```python
from build123d import *

# Parameters (mm, degrees)
F0_W         = 77.8764
F0_H         = 158.496
F1_DEPTH     = 7.2898
F2_R         = 9.525
F3_R         = 5.7077755574
F4_DEPTH     = 0.127
F5_W         = 9.2544863001
F5_H         = 0.6169676781
F6_DEPTH     = 0.381
F8_DEPTH     = 0.635
F9_R         = 1.016
F10_R        = 1.9930126565
F11_DEPTH    = 12.7
F13_W        = 8.6497310549
F13_H        = 2.2564521059
F14_DEPTH    = 12.7
F16_DEPTH    = 2.159
F18_DEPTH    = 0.635
F19_T1_DEPTH = 2.8833260431
F19_T3_DEPTH = 2.8575
F19_T5_DEPTH = 2.8319706152
F21_DEPTH    = 0.635
F22_T1_DEPTH = 3.4834715988
F22_T3_DEPTH = 3.4925
F22_T5_DEPTH = 3.5015570173
F23_R        = 0.635


# Not quite as in the source:
# - a fillet or chamfer that OpenCascade refuses, or shapes differently, is made with other operations: its cross-section is extruded or revolved along the edge and cut away or added


with BuildPart() as f1:
    # F0 (on Front) → F1 (new body)
    with BuildSketch(Plane.XZ):
        with Locations((-10.9280409528, 4.5388489962)):
            Rectangle(F0_W, F0_H)
    extrude(amount=F1_DEPTH)

    # F2
    f2_edges = [f1.edges().sort_by_distance(p)[0] for p in [
        (-49.866241, -3.6449, 83.786849),
        (28.010159, -3.6449, 83.786849),
        (28.010159, -3.6449, -74.709151),
        (-49.866241, -3.6449, -74.709151),
    ]]
    fillet(f2_edges, radius=F2_R)

    # F3 (on face) → F4 (cut)
    with BuildSketch(Plane.XZ.offset(7.2898)):
        with Locations((-9.174161778, -62.8947635373)):
            Circle(F3_R)
    extrude(amount=-F4_DEPTH, mode=Mode.SUBTRACT)

    # F5 (on face) → F6 (cut)
    with BuildSketch(Plane.XZ.offset(7.2898)):
        with Locations((-12.0077328756, 75.6440907717)):
            Rectangle(F5_W, F5_H)
    extrude(amount=-F6_DEPTH, mode=Mode.SUBTRACT)

    # F7 (on face) → F8 (join)
    with BuildSketch(Plane.YZ.offset(28.0101590472)):
        Polygon((-1.6678672982, 63.1312280893), (-5.6040398777, 63.1312280893), (-5.5761812255, 57.3286004364), (-1.6678672982, 57.3286004364), align=None)
    extrude(amount=F8_DEPTH)

    # F9
    f9_edges = [f1.edges().sort_by_distance(p)[0] for p in [
        (28.327659, -5.60404, 63.131228),
        (28.327659, -5.576181, 57.3286),
        (28.327659, -1.667867, 63.131228),
        (28.327659, -1.667867, 57.3286),
    ]]
    fillet(f9_edges, radius=F9_R)

    # F10 (on face) → F11 (cut)
    with BuildSketch(Plane(origin=(0, 0, -74.7091510038), x_dir=(1, 0, 0), z_dir=(0, 0, -1))):
        with Locations((-36.9087584466, 4.1701743638)):
            Circle(F10_R)
    extrude(amount=-F11_DEPTH, mode=Mode.SUBTRACT)

    # F13 (on face) → F14 (cut)
    with BuildSketch(Plane(origin=(0, 0, -74.7091510038), x_dir=(1, 0, 0), z_dir=(0, 0, -1))):
        with Locations((-8.9176273905, 3.8671875373)):
            Rectangle(F13_W, F13_H)
    extrude(amount=-F14_DEPTH, mode=Mode.SUBTRACT)

    # F15 (on face) → F16 (cut)
    with BuildSketch(Plane(origin=(-49.8662409528, 0, 0), x_dir=(0, -1, 0), z_dir=(-1, 0, 0))):
        Polygon((1.5233993763, 64.8115798831), (1.6149281291, 56.9802224636), (5.1021506079, 56.9802224636), (5.1021506079, 64.8115798831), align=None)
    extrude(amount=-F16_DEPTH, mode=Mode.SUBTRACT)

    # F17 (on face) → F18 (join)
    with BuildSketch(Plane(origin=(-49.8662409528, 0, 0), x_dir=(0, -1, 0), z_dir=(-1, 0, 0))):
        Polygon((2.3726914078, 50.4039227962), (2.4461376015, 44.0468862653), (4.1652750224, 44.0468862653), (4.1652750224, 50.4039227962), align=None)
    extrude(amount=F18_DEPTH)

    # F19: fillet of radius 0.889 on 4 edges, made by hand

    # F19_s2 → F19_t1 (cut)
    with BuildSketch(Plane.YZ.offset(-52.7495669959)):
        with BuildLine():
            ThreePointArc((-3.272021825, 50.4039227962), (-2.639783189, 50.1398990415), (-2.3830811527, 49.5046523961))
            Line((-2.3830811527, 49.5046523961), (-2.3726914078, 50.4039227962))
            Line((-2.3726914078, 50.4039227962), (-3.272021825, 50.4039227962))
        make_face()
    extrude(amount=F19_T1_DEPTH, mode=Mode.SUBTRACT)

    # F19_s4 → F19_t3 (cut)
    with BuildSketch(Plane.YZ.offset(-52.7237409528)):
        with BuildLine():
            ThreePointArc((-3.2762750224, 50.4039227962), (-3.9048929509, 50.1435407247), (-4.1652750224, 49.5149227962))
            Line((-4.1652750224, 49.5149227962), (-4.1652750224, 50.4039227962))
            Line((-4.1652750224, 50.4039227962), (-3.2762750224, 50.4039227962))
        make_face()
        with BuildLine():
            ThreePointArc((-4.1652750224, 44.9358862653), (-3.9048929509, 44.3072683368), (-3.2762750224, 44.0468862653))
            Line((-3.2762750224, 44.0468862653), (-4.1652750224, 44.0468862653))
            Line((-4.1652750224, 44.0468862653), (-4.1652750224, 44.9358862653))
        make_face()
    extrude(amount=F19_T3_DEPTH, mode=Mode.SUBTRACT)

    # F19_s6 → F19_t5 (cut)
    with BuildSketch(Plane.YZ.offset(-52.698211568)):
        with BuildLine():
            ThreePointArc((-3.3249258476, 44.0468862653), (-2.6999496023, 44.3036476293), (-2.4359851753, 44.9256158651))
            Line((-2.4359851753, 44.9256158651), (-2.4461376015, 44.0468862653))
            Line((-2.4461376015, 44.0468862653), (-3.3249258476, 44.0468862653))
        make_face()
    extrude(amount=F19_T5_DEPTH, mode=Mode.SUBTRACT)

    # F20 (on face) → F21 (join)
    with BuildSketch(Plane(origin=(-49.8662409528, 0, 0), x_dir=(0, -1, 0), z_dir=(-1, 0, 0))):
        Polygon((2.1069913637, 41.4195619524), (2.087448258, 35.2439321578), (3.8858172484, 35.2439321578), (3.8858172484, 41.4195619524), align=None)
    extrude(amount=F21_DEPTH)

    # F22: fillet of radius 1.143 on 4 edges, made by hand

    # F22_s2 → F22_t1 (cut)
    with BuildSketch(Plane.YZ.offset(-53.3497125516)):
        with BuildLine():
            ThreePointArc((-3.2463800032, 41.4195619524), (-2.4394367914, 41.0860628189), (-2.1033857264, 40.2801790179))
            Line((-2.1033857264, 40.2801790179), (-2.1069913637, 41.4195619524))
            Line((-2.1069913637, 41.4195619524), (-3.2463800032, 41.4195619524))
        make_face()
    extrude(amount=F22_T1_DEPTH, mode=Mode.SUBTRACT)

    # F22_s4 → F22_t3 (cut)
    with BuildSketch(Plane.YZ.offset(-53.3587409528)):
        with BuildLine():
            ThreePointArc((-2.7428172484, 41.4195619524), (-3.5510402993, 41.0847850032), (-3.8858172484, 40.2765619524))
            Line((-3.8858172484, 40.2765619524), (-3.8858172484, 41.4195619524))
            Line((-3.8858172484, 41.4195619524), (-2.7428172484, 41.4195619524))
        make_face()
        with BuildLine():
            ThreePointArc((-3.8858172484, 36.3869321578), (-3.5510402993, 35.5787091069), (-2.7428172484, 35.2439321578))
            Line((-2.7428172484, 35.2439321578), (-3.8858172484, 35.2439321578))
            Line((-3.8858172484, 35.2439321578), (-3.8858172484, 36.3869321578))
        make_face()
    extrude(amount=F22_T3_DEPTH, mode=Mode.SUBTRACT)

    # F22_s6 → F22_t5 (cut)
    with BuildSketch(Plane.YZ.offset(-53.3677979701)):
        with BuildLine():
            ThreePointArc((-3.2340710649, 35.2439321578), (-2.4245701983, 35.579988946), (-2.091076788, 36.3905492233))
            Line((-2.091076788, 36.3905492233), (-2.087448258, 35.2439321578))
            Line((-2.087448258, 35.2439321578), (-3.2340710649, 35.2439321578))
        make_face()
    extrude(amount=F22_T5_DEPTH, mode=Mode.SUBTRACT)

    # F23
    f23_edges = [f1.edges().sort_by_distance(p)[0] for p in [
        (-47.707241, -1.569164, 60.895901),
        (-47.707241, -3.358539, 56.980222),
        (-47.707241, -5.102151, 60.895901),
        (-47.707241, -3.312775, 64.81158),
        (-49.866241, -1.569164, 60.895901),
        (-48.786741, -5.102151, 56.980222),
        (-48.786741, -1.523399, 64.81158),
        (-49.866241, -5.102151, 60.895901),
        (-49.866241, -3.312775, 64.81158),
        (-49.866241, -3.358539, 56.980222),
    ]]
    fillet(f23_edges, radius=F23_R)


solid = f1.part
```
Check sheet for the modelled part. Datum: model origin and axes. Units: mm. A direction names the side the tool comes from. Give positions to 0.01 mm unless a question says otherwise; leave off trailing zeros. Order: outer loops, then holes, each group sorted by start corner. A loop starts at its lowest first (then second) coordinate and runs counter-clockwise, first axis right, second up. Notation, with made-up numbers: (5, 45.25) -> (19, 45.25) arc R16 ccw to (19, 74.25) -> close; hole circle Ø2 at (25, 5). An arc over 180 degrees is marked (long way). Use CSV: the item, a comma, the result in double quotes. Start each with the question number.
1) Mould release check, pull along Y, two halves, no side actions. Record for faces 1 (the face through (-38.49, -2.96, -68.45)), 2 (the face through (-11, 0, 6)), 3 (the face through (-11, -7.29, 6)), 4 (the face through (-47.15, -3.696, -71.845)): released by +Y, released by -Y, zero draft, split by the parting line, or undercut.
2) Sectioned sample at A-A, the plane z = -5. Record the boundary of the cut face in (x, y), plus the area to 3 significant figures.
3) Go/stop test with flat-tipped pins: P1, Ø5, axis at x = 19.5, z = 9.5, coming from the +Y side; P2, Ø1.1, axis at y = -4.5, z = -69.5, coming from the +X side; P3, Ø1, axis at x = -48.5, y = -3.5, coming from the +Z side; P4, Ø0.7, axis at x = 28.5, y = -3, coming from the -Z side. Record where each tip stops, or that it passes through.
4) Material ranges on line 1 (Z direction, x = -10, y = -7); line 2 (X direction, y = -3.5, z = -66); line 3 (X direction, y = -6.25, z = -32), recorded low to high. Write a range as from..to.
5) Set-up check for faces 5 (the face through (-9, -7.163, -63)), 6 (the face through (25.15, -3.7, -71.99)), 7 (the face through (-9, -2.739, -68)): record each of +Z, -Z, +X, -X, +Y, -Y from which the full face is reachable in a straight line by a thin tool's end or side.
Recorded:
1,face 1,"undercut"
1,face 2,"released by +Y"
1,face 3,"released by -Y"
1,face 4,"zero draft"
2,outline,"(-49.87, -7.29) -> (28.01, -7.29) -> (28.01, 0) -> (-49.87, 0) -> close"
2,area,"568 mm2"
3,P1,"y = 0"
3,P2,"x = 27.23"
3,P3,"z = 79.92"
3,P4,"z = 57.33"
4,line 1,"-74.71..75.34, 75.95..83.79"
4,line 2,"-49.83..-38.79, -35.03..-13.24, -4.59..27.98"
4,line 3,"-49.87..28.01"
5,face 5,"-Y"
5,face 6,"-Z, +X, +Y, -Y"
5,face 7,"-Z"
